from build123d import *

# Parameters (mm, degrees)
F1_DEPTH = 63.5
F2_DEPTH = 25.4
F3_DEPTH = 7.9375
F4_R     = 5.08


with BuildPart() as f1:
    # F0 (on Front) → F1 (new body, symmetric)
    with BuildSketch(Plane.XZ):
        Polygon((22.225, 9.525), (-41.275, 9.525), (-41.275, -9.525), (41.275, -9.525), (41.275, 9.525), align=None)
    extrude(amount=F1_DEPTH, both=True)

    # F0 (on Front) → F2 (join, symmetric)
    with BuildSketch(Plane.XZ):
        with BuildLine():
            Line((22.225, 27.0002), (22.225, 9.525))
            Line((22.225, 9.525), (41.275, 9.525))
            Line((41.275, 9.525), (41.275, 27.0002))
            ThreePointArc((41.275, 27.0002), (45.92468, 38.22552), (57.15, 42.8752))
            Line((57.15, 42.8752), (60.325, 42.8752))
            Line((60.325, 42.8752), (60.325, 61.9252))
            Line((60.325, 61.9252), (57.15, 61.9252))
            ThreePointArc((57.15, 61.9252), (32.454296, 51.695904), (22.225, 27.0002))
        make_face()
        Polygon((60.325, 66.675), (60.325, 61.9252), (60.325, 42.8752), (60.325, 38.1), (111.125, 38.1), (111.125, 66.675), align=None)
    extrude(amount=F2_DEPTH, both=True)

    # F0 (on Front) → F3 (join, symmetric)
    with BuildSketch(Plane.XZ):
        with BuildLine():
            add(Edge.make_bspline(
                [(-41.275, 9.525), (-42.032037, 59.136383), (12.069872, 61.952318), (57.15, 61.9252)],
                knots=[0, 0, 0, 0, 111.504536, 111.504536, 111.504536, 111.504536], degree=3))
            Line((-41.275, 9.525), (22.225, 9.525))
            Line((22.225, 9.525), (22.225, 27.0002))
            ThreePointArc((22.225, 27.0002), (32.454296, 51.695904), (57.15, 61.9252))
        make_face()
    extrude(amount=F3_DEPTH, both=True)

    # F4
    f4_edges = [f1.edges().sort_by_distance(p)[0] for p in [
        (-41.275, -63.5, 0),
        (41.275, -63.5, 0),
        (41.275, 63.5, 0),
        (-41.275, 63.5, 0),
    ]]
    fillet(f4_edges, radius=F4_R)


solid = f1.part
Model file for the job. Use its own axes, mm. A direction names the side the tool comes from. Give positions to 0.01 mm unless a question says otherwise; leave off trailing zeros. Order: outer loops, then holes, each group sorted by start corner. A loop starts at its lowest first (then second) coordinate and runs counter-clockwise, first axis right, second up. Notation, with made-up numbers: M 81,-2 L 123,-2 A24 cw 123,13 Z; hole C 84.25,-37 d11. An arc over 180 degrees is marked long. Put each result on its own line as item: value. Start each with the question number.
(1) Pin check, flat tips, straight feed: pin 1 Ø3 at (x, z) = (-9, 36.5) entering from -Y; pin 2 Ø12 at (x, z) = (68.5, 53) entering from +Y; pin 3 Ø2.5 at (x, y) = (59, 1) entering from +Z. Stop position of each tip, or through.
(2) Band-saw the part on A-A on y = -20. Give the cut face in (x, z) (3 decimals), then the cut area to 3 significant figures.
(3) Band-saw the part on D-D on y = 38.5. Give the cut face in (x, z) (3 decimals), then the cut area to 3 significant figures.
(4) Tool access for faces 1 (the face through (60.325, 0, 41)), 2 (the face through (32.73, 16.55, 51.97)), 3 (the face through (22.225, -17, 18)): list every direction of +Z, -Z, +X, -X, +Y, -Y with a clear straight run to the whole face (end or side of a thin tool).
(5) Band-saw the part on B-B on z = -3.5. Give the cut face in (x, y) (3 decimals).
(6) Band-saw the part on C-C on x = 84. Give the cut face in (y, z) (3 decimals), then the cut area to 3 significant figures.
(7) Drill centre lines: L1, parallel to X at y = -30, z = -4 (3 decimals); L2, parallel to Y at x = -17, z = 33; L3, parallel to Z at x = 56, y = 10.5. Where is each one in solid material? Low to high. Write a range as [from, to].
(8) Pull direction X, two halves, no side cores. Call faces 4 (the face through (45.8, -0.4, 38.1)), 5 (the face through (32.73, -16.79, 51.97)), 6 (the face through (-3, 7.938, 30)): released by +X, released by -X, zero draft, split by the parting line, or undercut.
Results below:
1. pin 1: stops at y = -7.94
1. pin 2: stops at y = 25.4
1. pin 3: stops at z = 61.93
2. outline: M -41.275,-9.525 L 41.275,-9.525 L 41.275,27 A15.875 cw 57.15,42.875 L 60.325,42.875 L 60.325,38.1 L 111.125,38.1 L 111.125,66.675 L 60.325,66.675 L 60.325,61.925 L 57.15,61.925 A34.925 ccw 22.225,27 L 22.225,9.525 L -41.275,9.525 Z
2. area: 4,180 mm2
3. outline: M -41.275,-9.525 L 41.275,-9.525 L 41.275,9.525 L -41.275,9.525 Z
3. area: 1,570 mm2
4. face 1: -Z, +Y, -Y
4. face 2: +Z, -X, +Y
4. face 3: +Z, -X, -Y
5. outline: M -41.275,-58.42 A5.08 ccw -36.195,-63.5 L 36.195,-63.5 A5.08 ccw 41.275,-58.42 L 41.275,58.42 A5.08 ccw 36.195,63.5 L -36.195,63.5 A5.08 ccw -41.275,58.42 Z
6. outline: M -25.4,38.1 L 25.4,38.1 L 25.4,66.675 L -25.4,66.675 Z
6. area: 1,450 mm2
7. L1: x = [-41.275, 41.275]
7. L2: y = [-7.94, 7.94]
7. L3: z = [42.83, 61.91]
8. face 4: undercut
8. face 5: released by -X
8. face 6: zero draft
